Read the model definition and answer for the solid it produces. Units are mm, in the model's axes. Face numbers are marked on the shaded views. A direction names the side the tool comes from. Coordinates: 2 decimals unless noted, no trailing zeros. Write each loop counter-clockwise with the first axis right and the second up, starting at its lowest first coordinate (ties: lowest second). Pieces come first, ordered by that corner, then holes. Notation, with made-up numbers: (60.5, -36.75) -> (68.5, -36.75) arc R21 ccw to (68.5, -29.75) -> close; hole circle Ø8 at (80, 14.5). An arc over 180 degrees is marked (long way). One line per item, written item: value. Start each with the question number.
from build123d import *

# Parameters (mm, degrees)
SKETCH2_W                      = 516
SKETCH2_H                      = 198
SKETCH2_W_2                    = 65
SKETCH2_H_2                    = 178
SKETCH2_W_3                    = 416
BOSS_EXTRUDE2_DEPTH            = 45
DRAFT3_ANGLE                   = 20
FILLET1_R                      = 10
SKETCH2_3_W                    = 416
SKETCH2_3_H                    = 178
SKETCH2_3_W_2                  = 350
SKETCH2_3_H_2                  = 80
SKETCH2_3_W_3                  = 376
SKETCH2_3_H_3                  = 68
SKETCH2_3_W_4                  = 65
BOSS_EXTRUDE3_DEPTH            = 2
CUT_EXTRUDE1_DEPTH             = 5
CUT_EXTRUDE2_REACH             = 538.858
SKETCH4_R                      = 10
CUT_EXTRUDE2_DIRECTION_2_DEPTH = 54
SKETCH5_R                      = 7.5
CUT_EXTRUDE3_DEPTH             = 15


with BuildPart() as part:
    # Sketch2 → Boss-Extrude2 (new body)
    with BuildSketch(Plane(origin=(0, 0, 0), x_dir=(1, 0, 0), z_dir=(0, 1, 0))):
        Rectangle(SKETCH2_W, SKETCH2_H)
        with Locations((215.5, 0)):
            Rectangle(SKETCH2_W_2, SKETCH2_H_2, mode=Mode.SUBTRACT)
        with Locations((-40, 0)):
            Rectangle(SKETCH2_W_3, SKETCH2_H_2, mode=Mode.SUBTRACT)
    extrude(amount=BOSS_EXTRUDE2_DEPTH)

    # Draft3
    draft3_faces = [part.faces().sort_by_distance(p)[0] for p in [
        (0, 22.5, -99),
        (258, 22.5, 0),
        (0, 22.5, 99),
        (-258, 22.5, 0),
    ]]
    draft(draft3_faces, Plane.ZX.offset(45), DRAFT3_ANGLE)

    # Fillet1
    fillet1_edges = [part.edges().sort_by_distance(p)[0] for p in [
        (-248, 22.5, 89),
        (168, 22.5, 89),
        (168, 22.5, -89),
        (-248, 22.5, -89),
        (-266.189330271, 22.5, -107.189330271),
        (266.189330271, 22.5, -107.189330271),
        (266.189330271, 22.5, 107.189330271),
        (-266.189330271, 22.5, 107.189330271),
        (248, 22.5, 89),
        (248, 22.5, -89),
        (183, 22.5, -89),
        (183, 22.5, 89),
    ]]
    fillet(fillet1_edges, radius=FILLET1_R)

    # Sketch2<3> → Boss-Extrude3 (add)
    # profile 1 of 4: a face of its own
    with BuildSketch(Plane(origin=(0, 0, 0), x_dir=(1, 0, 0), z_dir=(0, 1, 0))):
        with Locations((-40, 0)):
            Rectangle(SKETCH2_3_W, SKETCH2_3_H)
        with Locations((-63, 44)):
            Rectangle(SKETCH2_3_W_2, SKETCH2_3_H_2, mode=Mode.SUBTRACT)
        with Locations((-50, -45)):
            Rectangle(SKETCH2_3_W_3, SKETCH2_3_H_3, mode=Mode.SUBTRACT)
    # profile 2 of 4: a face of its own
    with BuildSketch(Plane(origin=(0, 0, 0), x_dir=(1, 0, 0), z_dir=(0, 1, 0))):
        with Locations((-50, -45)):
            Rectangle(SKETCH2_3_W_3, SKETCH2_3_H_3)
    # profile 3 of 4: a face of its own
    with BuildSketch(Plane(origin=(0, 0, 0), x_dir=(1, 0, 0), z_dir=(0, 1, 0))):
        with Locations((-63, 44)):
            Rectangle(SKETCH2_3_W_2, SKETCH2_3_H_2)
    # profile 4 of 4: a face of its own
    with BuildSketch(Plane(origin=(0, 0, 0), x_dir=(1, 0, 0), z_dir=(0, 1, 0))):
        with Locations((215.5, 0)):
            Rectangle(SKETCH2_3_W_4, SKETCH2_3_H)
    extrude(amount=BOSS_EXTRUDE3_DEPTH)

    # Sketch3 → Cut-Extrude1 (cut)
    with BuildSketch(Plane(origin=(0, 45, 0), x_dir=(1, 0, 0), z_dir=(0, 1, 0))):
        with BuildLine():
            Line((171, -79), (171, 79))
            ThreePointArc((171, 79), (167.192388155, 88.192388155), (158, 92))
            Line((158, 92), (-238, 92))
            ThreePointArc((-238, 92), (-247.192388155, 88.192388155), (-251, 79))
            Line((-251, 79), (-251, -79))
            ThreePointArc((-251, -79), (-247.192388155, -88.192388155), (-238, -92))
            Line((-238, -92), (158, -92))
            ThreePointArc((158, -92), (167.192388155, -88.192388155), (171, -79))
        make_face()
        with BuildLine():
            Line((193, -92), (238, -92))
            ThreePointArc((238, -92), (247.192388155, -88.192388155), (251, -79))
            Line((251, -79), (251, 79))
            ThreePointArc((251, 79), (247.192388155, 88.192388155), (238, 92))
            Line((238, 92), (193, 92))
            ThreePointArc((193, 92), (183.807611845, 88.192388155), (180, 79))
            Line((180, 79), (180, -79))
            ThreePointArc((180, -79), (183.807611845, -88.192388155), (193, -92))
        make_face()
    extrude(amount=-CUT_EXTRUDE1_DEPTH, mode=Mode.SUBTRACT)

    # Cut-Extrude2: up to this face of the body (flat: up to its plane)
    cut_extrude2_end = Plane(part.part.faces().sort_by_distance((168, 21, 0))[0])
    # Sketch4 → Cut-Extrude2 (cut, up to the picked face)
    with BuildSketch(Plane.ZY.offset(-248), mode=Mode.PRIVATE) as cut_extrude2_sk1:
        with Locations((-39, 21)):
            Circle(SKETCH4_R)
    cut_extrude2_tool1 = split(extrude(cut_extrude2_sk1.sketch, amount=CUT_EXTRUDE2_REACH, mode=Mode.PRIVATE), bisect_by=cut_extrude2_end, keep=Keep.BOTH, mode=Mode.PRIVATE)
    add(cut_extrude2_tool1.solids().sort_by(Axis((248, 21, -39), (-1, 0, 0)))[0], mode=Mode.SUBTRACT)

    # Sketch4 → Cut-Extrude2 direction 2 (cut)
    with BuildSketch(Plane.ZY.offset(-248)):
        with Locations((-39, 21)):
            Circle(SKETCH4_R)
    extrude(amount=-CUT_EXTRUDE2_DIRECTION_2_DEPTH, mode=Mode.SUBTRACT)

    # Sketch5 → Cut-Extrude3 (cut)
    with BuildSketch(Plane(origin=(183, 0, 0), x_dir=(0, 0, -1), z_dir=(1, 0, 0))):
        with Locations((-29, 21)):
            Circle(SKETCH5_R)
    extrude(amount=-CUT_EXTRUDE3_DEPTH, mode=Mode.SUBTRACT)


solid = part.part
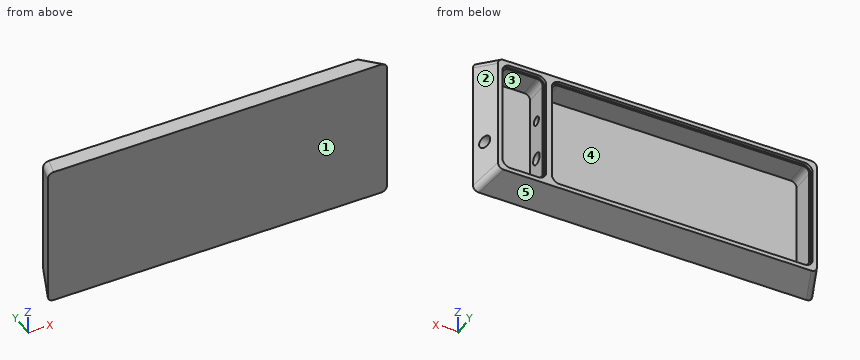
1. Given pin 1 (2.5 mm diameter, centred on x = 10.5, y = 41.5, fed in from -Z); pin 2 (2 mm diameter, centred on x = -181, y = 15.5, fed in from -Z); pin 3 (1 mm diameter, centred on y = 40, z = -83.5, fed in from -X), each flat-ended and moving along its own axis, determine where each tip first touches the part or whether it passes through.
2. Find the intervals of material crossed by probe 1 along X at (y, z) = (26, -1.5); probe 2 along X at (y, z) = (24.5, -23.5); probe 3 along Y at (x, z) = (178, 29), in increasing order. Write a range as from..to.
3. A cutting plane is placed at B-B on z = 53. Give the vertices of the cut face in (x, y).
4. A cutting plane is placed at A-A on z = 29. Give the vertices of the cut face in (x, y).
5. A cutting plane is placed at D-D on z = -39. Give the vertices of the cut face in (x, y), then the cut area to 3 significant figures.
6. A tool of negligible diameter and unlimited length cuts with its end or side. For the marked faces 4 and 5, from which of +Z, -Z, +X, -X, +Y, -Y can it reach the whole face along a straight path? Write none if from no direction.
7. For a pull along X with two mould halves and no side action, classify the marked faces 1, 2 and 3 as +X half, -X half, draft (parallel to the pull), parting line (faces both ways), or undercut.
8. A cutting plane is placed at C-C on x = 67.5. Give the vertices of the cut face in (y, z).
Derived:
1. pin 1: stops at z = -100.73
1. pin 2: stops at z = -110.1
1. pin 3: stops at x = -260
2. probe 1: x = -264.92..-248, 168..183, 248..264.92
2. probe 2: x = -265.46..-248, 168..183, 248..265.46
2. probe 3: y = 0..13.5, 28.5..45
3. outline: (-274.38, 0) -> (274.38, 0) -> (258, 45) -> (251, 45) -> (251, 40) -> (248, 40) -> (248, 2) -> (183, 2) -> (183, 40) -> (180, 40) -> (180, 45) -> (171, 45) -> (171, 40) -> (168, 40) -> (168, 2) -> (-248, 2) -> (-248, 40) -> (-251, 40) -> (-251, 45) -> (-258, 45) -> close
4. outline: (-274.38, 0) -> (274.38, 0) -> (258, 45) -> (251, 45) -> (251, 40) -> (248, 40) -> (248, 2) -> (183, 2) -> (183, 13.5) -> (168, 13.5) -> (168, 2) -> (-248, 2) -> (-248, 40) -> (-251, 40) -> (-251, 45) -> (-258, 45) -> close; (168, 28.5) -> (183, 28.5) -> (183, 40) -> (180, 40) -> (180, 45) -> (171, 45) -> (171, 40) -> (168, 40) -> close
5. outline: (-274.38, 0) -> (274.38, 0) -> (270.37, 11) -> (248, 11) -> (248, 2) -> (183, 2) -> (183, 11) -> (168, 11) -> (168, 2) -> (-248, 2) -> (-248, 40) -> (-251, 40) -> (-251, 45) -> (-258, 45) -> close; (168, 31) -> (183, 31) -> (183, 40) -> (180, 40) -> (180, 45) -> (171, 45) -> (171, 40) -> (168, 40) -> close; (248, 31) -> (263.1, 31) -> (258, 45) -> (251, 45) -> (251, 40) -> (248, 40) -> close
5. area: 2,540 mm2
6. face 4: +Y
6. face 5: -Z, +X, -X, +Y
7. face 1: draft
7. face 2: +X half
7. face 3: undercut
8. outline: (0, -115.38) -> (45, -99) -> (45, -92) -> (40, -92) -> (40, -89) -> (2, -89) -> (2, 89) -> (40, 89) -> (40, 92) -> (45, 92) -> (45, 99) -> (0, 115.38) -> close
